Autodesk Inventor part; units mm, degrees
ref_plane "YZ Plane" through (0, 0, 0) normal (1, 0, 0) x (0, 1, 0)
ref_plane "XZ Plane" through (0, 0, 0) normal (0, 1, 0) x (-1, 0, 0)
ref_plane "XY Plane" through (0, 0, 0) normal (0, 0, 1) x (1, 0, 0)
sketch "スケッチ1" plane through (0, 0, 0) normal (0, 0, 1) x (1, 0, 0)
  line L0 (-17.5, 17.5) -> (17.5, 17.5)
  line L1 (17.5, 17.5) -> (17.5, -17.5)
  line L2 (17.5, -17.5) -> (-17.5, -17.5)
  line L3 (-17.5, -17.5) -> (-17.5, 17.5)
  point P0 (0, 0)
  dimension "d0" = 35
  dimension "d1" = 35
  dimension "d2" = 17.5
  dimension "d3" = 17.5
extrude "押し出し1" add sketch "スケッチ1" along normal blind 7
sketch "スケッチ2" plane through (0, 0, 7) normal (0, 0, 1) x (1, 0, 0)
  line L0 (-17.5, 17.5) -> (17.5, -17.5)
  line L1 (17.5, 17.5) -> (-17.5, -17.5)
  line L2 (-17.5, -17.5) -> (-17.5, 17.5)
  circle A0 centre (0, 0) radius 18.5
  point P0 (-13.0815, 13.0815)
  point P1 (13.0815, 13.0815)
  point P2 (13.0815, -13.0815)
  point P3 (-13.0815, -13.0815)
  dimension "d6" = 37
hole "Hole1" at (-13.0815, 13.0815, 7) at (13.0815, 13.0815, 7) at (13.0815, -13.0815, 7) at (-13.0815, -13.0815, 7) direction (0, 0, -1) diameter 2 end through all
sketch "スケッチ3" plane through (0, 0, 7) normal (0, 0, 1) x (1, 0, 0)
  circle A0 centre (0, 0) radius 7.5
  circle A1 centre (0, 0) radius 6.5
  dimension "d14" = 15
  dimension "d15" = 13
extrude "押し出し2" add sketch "スケッチ3" along normal blind 2
sketch "スケッチ4" plane through (0, 0, 7) normal (0, 0, 1) x (1, 0, 0)
  line L0 (17.5, 17.5) -> (17.5, -17.5)
  line L1 (-17.5, 17.5) -> (17.5, 17.5)
  line L2 (-17.5, -17.5) -> (-17.5, 17.5)
  line L3 (17.5, -17.5) -> (-17.5, -17.5)
  line L4 (17.5, 13.5) -> (15.5, 13.5)
  line L5 (15.5, 13.5) -> (15.5, 9.9)
  line L6 (15.5, 9.9) -> (17.5, 9.9)
  line L7 (17.5, 9.9) -> (17.5, 13.5)
  line L8 (17.5, 0) -> (-17.5, 0)
  line L9 (17.5, -17.5) -> (17.5, 17.5)
  line L10 (17.5, -13.5) -> (15.5, -13.5)
  line L11 (15.5, -13.5) -> (15.5, -9.9)
  line L12 (15.5, -9.9) -> (17.5, -9.9)
  line L13 (17.5, -9.9) -> (17.5, -13.5)
  line L14 (0, 17.5) -> (0, -17.5)
  line L15 (-17.5, 17.5) -> (-17.5, -17.5)
  line L16 (-17.5, 13.5) -> (-15.5, 13.5)
  line L17 (-15.5, 13.5) -> (-15.5, 9.9)
  line L18 (-15.5, 9.9) -> (-17.5, 9.9)
  line L19 (-17.5, 9.9) -> (-17.5, 13.5)
  line L20 (-17.5, -17.5) -> (-17.5, 17.5)
  line L21 (-15.5, -13.5) -> (-15.5, -9.9)
  line L22 (-15.5, -9.9) -> (-17.5, -9.9)
  line L23 (-17.5, -9.9) -> (-17.5, -13.5)
  line L24 (-17.5, -13.5) -> (-15.5, -13.5)
  dimension "d18" = 4
  dimension "d19" = 2
  dimension "d20" = 3.6
extrude "押し出し3" cut sketch "スケッチ4" against normal blind 2 contours L0 L6 L5 L4 | L16 L17 L18 L2 | L0 L10 L11 L12 | L22 L21 L24 L2
sketch "スケッチ5" plane through (0, 0, 0) normal (0, 0, -1) x (-1, 0, 0)
  line L0 (17.5, 17.5) -> (-17.5, 17.5)
  line L1 (-17.5, 17.5) -> (-17.5, -17.5)
  line L2 (-17.5, -17.5) -> (17.5, -17.5)
  line L3 (17.5, 0) -> (-17.5, 0)
  line L4 (17.5, 17.5) -> (-17.5, 17.5)
  line L5 (0, 17.5) -> (0, -17.5)
  line L6 (15.5, 13.5) -> (17, 13.5)
  line L7 (17, 13.5) -> (17, 9.9)
  line L8 (17, 9.9) -> (15.5, 9.9)
  line L9 (15.5, 9.9) -> (15.5, 13.5)
  line L10 (17.5, -17.5) -> (17.5, 17.5)
  line L11 (15.5, -13.5) -> (17, -13.5)
  line L12 (17, -13.5) -> (17, -9.9)
  line L13 (17, -9.9) -> (15.5, -9.9)
  line L14 (15.5, -9.9) -> (15.5, -13.5)
  line L15 (-15.5, 13.5) -> (-17, 13.5)
  line L16 (-17, 13.5) -> (-17, 9.9)
  line L17 (-17, 9.9) -> (-15.5, 9.9)
  line L18 (-15.5, 9.9) -> (-15.5, 13.5)
  line L19 (-15.5, -13.5) -> (-17, -13.5)
  line L20 (-17, -13.5) -> (-17, -9.9)
  line L21 (-17, -9.9) -> (-15.5, -9.9)
  line L22 (-15.5, -9.9) -> (-15.5, -13.5)
  line L23 (17, 13.5) -> (15.5, 13.5)
  line L24 (15.5, 13.5) -> (15.5, 9.9)
  line L25 (15.5, 9.9) -> (17, 9.9)
  line L26 (17, 9.9) -> (17, 13.5)
  point P0 (0, 0)
  dimension "d26" = 4
  dimension "d27" = 3.6
  dimension "d28" = 2
  dimension "d29" = 1.5
extrude "押し出し4" cut sketch "スケッチ5" against normal through all contours L6 L7 L8 L9 | L14 L13 L12 L11 | L18 L17 L16 L15 | L19 L20 L21 L22
sketch "スケッチ6" plane through (-17.5, -17.5, 0) normal (-1, 0, 0) x (0, 0, 1)
  line L0 (0, 0) -> (0, 35)
  line L1 (0, 35) -> (0, 0)
  line L2 (2, 31) -> (0, 31)
  line L3 (0, 31) -> (0, 30.7)
  line L4 (0, 30.7) -> (2, 30.7)
  line L5 (2, 30.7) -> (2, 31)
  line L6 (2, 27.4) -> (0, 27.4)
  line L7 (0, 27.4) -> (0, 27.7)
  line L8 (0, 27.7) -> (2, 27.7)
  line L9 (2, 27.7) -> (2, 27.4)
  line L10 (7, 27.4) -> (7, 7.6)
  line L11 (7, 17.5) -> (0, 17.5)
  line L12 (0, 0) -> (0, 35)
  line L13 (2, 4) -> (0, 4)
  line L14 (0, 4) -> (0, 4.3)
  line L15 (0, 4.3) -> (2, 4.3)
  line L16 (2, 4.3) -> (2, 4)
  line L17 (2, 7.6) -> (0, 7.6)
  line L18 (0, 7.6) -> (0, 7.3)
  line L19 (0, 7.3) -> (2, 7.3)
  line L20 (2, 7.3) -> (2, 7.6)
  dimension "d32" = 3
  dimension "d33" = 0.3
  dimension "d34" = 2
extrude "押し出し5" cut sketch "スケッチ6" against normal blind 2
sketch "スケッチ7" plane through (17.5, -17.5, 0) normal (1, 0, 0) x (0, 0, -1)
  line L0 (-7, 27.4) -> (-7, 7.6)
  line L1 (-7, 17.5) -> (0, 17.5)
  line L2 (-2, 4.3) -> (0, 4.3)
  line L3 (0, 4.3) -> (0, 4)
  line L4 (0, 4) -> (-2, 4)
  line L5 (-2, 4) -> (-2, 4.3)
  line L6 (-2, 27.4) -> (0, 27.4)
  line L7 (0, 27.4) -> (0, 27.7)
  line L8 (0, 27.7) -> (-2, 27.7)
  line L9 (-2, 27.7) -> (-2, 27.4)
  line L10 (-2, 31) -> (0, 31)
  line L11 (0, 31) -> (0, 30.7)
  line L12 (0, 30.7) -> (-2, 30.7)
  line L13 (-2, 30.7) -> (-2, 31)
  line L14 (0, 7.6) -> (-2, 7.6)
  line L15 (-2, 7.6) -> (-2, 7.3)
  line L16 (-2, 7.3) -> (0, 7.3)
  line L17 (0, 7.3) -> (0, 7.6)
  dimension "d40" = 0.3
extrude "押し出し6" cut sketch "スケッチ7" against normal blind 2
sketch "スケッチ8" plane through (0, 0, 0) normal (0, 0, -1) x (-1, 0, 0)
  line L0 (-17, 13.2) -> (-17.5, 13.2)
  line L1 (-17.5, 13.2) -> (-17.5, 10.2)
  line L2 (-17.5, 10.2) -> (-17, 10.2)
  line L3 (-17, 10.2) -> (-17, 13.2)
  point P0 (0, 0)
extrude "押し出し7" add sketch "スケッチ8" along normal blind 2
sketch "スケッチ9" plane through (0, 0, 0) normal (0, 0, -1) x (-1, 0, 0)
  line L0 (-17, -10.2) -> (-17.5, -10.2)
  line L1 (-17.5, -10.2) -> (-17.5, -13.2)
  line L2 (-17.5, -13.2) -> (-17, -13.2)
  line L3 (-17, -13.2) -> (-17, -10.2)
  point P0 (0, 0)
extrude "押し出し8" add sketch "スケッチ9" along normal blind 2
sketch "スケッチ10" plane through (0, 0, 0) normal (0, 0, -1) x (-1, 0, 0)
  line L0 (17, -13.2) -> (17.5, -13.2)
  line L1 (17.5, -13.2) -> (17.5, -10.2)
  line L2 (17.5, -10.2) -> (17, -10.2)
  line L3 (17, -10.2) -> (17, -13.2)
  point P0 (0, 0)
extrude "押し出し9" add sketch "スケッチ10" along normal blind 2
sketch "スケッチ11" plane through (0, 0, 0) normal (0, 0, -1) x (-1, 0, 0)
  line L0 (17.5, 13.2) -> (17, 13.2)
  line L1 (17, 13.2) -> (17, 10.2)
  line L2 (17, 10.2) -> (17.5, 10.2)
  line L3 (17.5, 10.2) -> (17.5, 13.2)
  point P0 (0, 0)
extrude "押し出し10" add sketch "スケッチ11" along normal blind 2
fillet "フィレット2" radius 1.5 4 edges at (17.5, -17.5, 3.5) (-17.5, -17.5, 3.5) (-17.5, 17.5, 3.5) (17.5, 17.5, 3.5)
sketch "スケッチ14" plane through (0, 0, 7) normal (0, 0, 1) x (1, 0, 0)
  circle A0 centre (0, 0) radius 6.5
hole "Hole3" at (0, 0, 7) direction (0, 0, -1) diameter 6.5 end through all
equation "\"d1\" = d0"
properties part number "SLIPRING_SRG-1-6G"
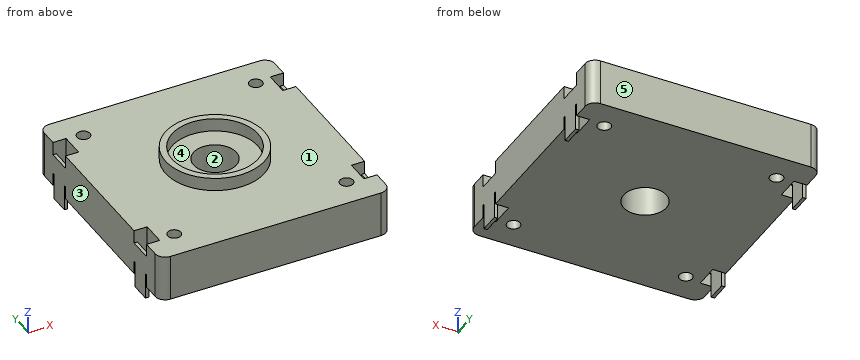
CAD build for the part. Positions are in the model's coordinates, mm. Face numbers are marked on the shaded views. A direction names the side the tool comes from. Give positions to 0.01 mm unless a question says otherwise; leave off trailing zeros. Write each loop counter-clockwise with the first axis right and the second up, starting at its lowest first coordinate (ties: lowest second). Pieces come first, ordered by that corner, then holes. Notation, with made-up numbers: (51, -32) - (56, -32) arc R5 cw to (56, -25) - close; hole circle Ø6 at (39.5, 17.5). An arc over 180 degrees is marked (long way). Put each result on its own line as item: value.
(1) Tool access for the marked faces 4 and 5: list every direction of +Z, -Z, +X, -X, +Y, -Y with a clear straight run to the whole face (end or side of a thin tool).
Working result:
face 4: +Z
face 5: +Z, -Z, +X, -X, +Y
(2) Saw through at C-C (x = 0). List the corners of the cut face in (y, z), then the cut area to 4 significant figures.
Working result:
outline: (-17.5, 0) - (-3.25, 0) - (-3.25, 7) - (-6.5, 7) - (-6.5, 9) - (-7.5, 9) - (-7.5, 7) - (-17.5, 7) - close; (3.25, 0) - (17.5, 0) - (17.5, 7) - (7.5, 7) - (7.5, 9) - (6.5, 9) - (6.5, 7) - (3.25, 7) - close
area: 203.5 mm^2
(3) Saw through at A-A (y = -11). List the corners of the cut face in (x, z).
Working result:
outline: (-17.5, -2) - (-17, -2) - (-17, 5) - (-17.5, 5) - close; (-15.5, 0) - (15.5, 0) - (15.5, 7) - (-15.5, 7) - close; (17, -2) - (17.5, -2) - (17.5, 5) - (17, 5) - close
(4) Saw through at B-B (z = -1). List the corners of the cut face in (x, y), then the cut area to 3 significant figures.
Working result:
outline: (-17.5, -13.2) - (-17, -13.2) - (-17, -10.2) - (-17.5, -10.2) - close; (-17.5, 10.2) - (-17, 10.2) - (-17, 13.2) - (-17.5, 13.2) - close; (17, -13.2) - (17.5, -13.2) - (17.5, -10.2) - (17, -10.2) - close; (17, 10.2) - (17.5, 10.2) - (17.5, 13.2) - (17, 13.2) - close
area: 6.00 mm^2
(5) Pull direction X, two halves, no side cores. Call the marked faces 1, 2 and 3: released by +X, released by -X, zero draft, split by the parting line, or undercut.
Working result:
face 1: zero draft
face 2: undercut
face 3: released by -X
(6) Drop flat-ended pins along their axis: pin 1 Ø1 at (x, z) = (16.5, 2) entering from -Y; pin 2 Ø3 at (x, y) = (-13.08, 13.08) entering from -Z; pin 3 Ø3 at (x, y) = (2.5, 13) entering from +Z; pin 4 Ø1.6 at (x, z) = (-17, 3.5) entering from +Y. Give the stop position or say it passes through.
Working result:
pin 1: y = -17.5
pin 2: z = 0
pin 3: z = 7
pin 4: y = 17.49
(7) Wall check: L1, parallel to X at y = -13, z = 6.5; L2, parallel to Y at x = -13, z = 0.75; L3, parallel to X at y = -11, z = 2.25. Give the ranges that are in metal, low to high.
Working result:
L1: -15.5 to -14.08, -12.08 to 12.08, 14.08 to 15.5
L2: -17.5 to -14.08, -12.08 to 12.08, 14.08 to 17.5
L3: -17.5 to -17, -15.5 to 15.5, 17 to 17.5
